Design review of the part built by this model. Coordinates are the model's own, in mm. A direction names the side the tool comes from. Give positions to 0.01 mm unless a question says otherwise; leave off trailing zeros. Write each loop counter-clockwise with the first axis right and the second up, starting at its lowest first coordinate (ties: lowest second). Pieces come first, ordered by that corner, then holes. Notation, with made-up numbers: (-0.75, 41) -> (32.25, 41) arc R22 ccw to (32.25, 67) -> close; hole circle Ø11 at (80.5, 68). An arc over 180 degrees is marked (long way). Write each question's results on one line, items separated by ' | '. Start each with the question number.
(1) Take a section at D-D (x = -28). State the section outline as (y, z) points (3 decimals).
(2) To check wall thickness, follow probe 1 along Z at (x, y) = (-16.5, -0.7); probe 2 along Z at (x, y) = (-2, -0.65); probe 3 along X at (y, z) = (-0.5, -3). State the ranges of each line that lie inside material, in increasing order.
(3) Mouldability with a two-part tool opening along Z and no side actions: class faces 3 (the face through (6, -3.175, -3)), 4 (the face through (-8.774, -1.565, -53.198)), 5 (the face through (-5.525, -1.565, 3.131)) as released by +Z, released by -Z, zero draft, split by the parting line, or undercut.
(4) Clearance check with flat-ended pins moving along their axes: pin 1 (1 mm diameter, centred on x = 24, y = -1.5, fed in from -Z); pin 2 (1 mm diameter, centred on x = -1.5, y = -2, fed in from +Z); pin 3 (6 mm diameter, centred on x = -46, z = 6.5, fed in from +Y). State where each tip first meets the part, or that it passes through.
(5) For faces 1 (the face through (5.474, -1.565, 3.219)), 2 (the face through (6, 0, -3)), list the 3-axis set-ups (+Z, -Z, +X, -X, +Y, -Y) from which the entire face can be reached by the end or side of a thin tool; tool diameter is ignored.
(6) Take a section at B-B (z = -13). State the section outline as (x, y) points (3 decimals), plus the area to 3 significant figures.
(7) Take a section at A-A (y = -2.2). State the section outline as (x, z) points, plus the area to 3 significant figures.
(8) Take a section at C-C (z = 18). State the section outline as (x, y) points (3 decimals), plus the area to 3 significant figures.
from build123d import *

# Parameters (mm, degrees)
F1_DEPTH = 3.175


with BuildPart() as f1:
    # F0 (on Front) → F1 (new body)
    with BuildSketch(Plane.XZ):
        with BuildLine():
            ThreePointArc((32.9955675162, -19.0500006373), (36.8017738864, -9.8610059738), (38.1, 0))
            ThreePointArc((38.1, 0), (26.9407683703, 26.9407683561), (2.01e-08, 38.1))
            ThreePointArc((2.01e-08, 38.1), (-32.9955680289, 19.0499997494), (-32.9955675847, -19.0500005187))
            ThreePointArc((-32.9955675847, -19.0500005187), (-6.85e-08, -38.1), (32.9955675162, -19.0500006373))
        make_face()
        Polygon((3.6661742094, 6.35), (7.3323484187, 0), (3.6661742094, -6.35), (-3.6661742094, -6.35), (-7.3323484187, 0), (-3.6661742094, 6.35), align=None, mode=Mode.SUBTRACT)
        with BuildLine():
            ThreePointArc((2.01e-08, 38.1), (26.9407683703, 26.9407683561), (38.1, 0))
            ThreePointArc((38.1, 0), (36.8017738864, -9.8610059738), (32.9955675162, -19.0500006373))
            ThreePointArc((32.9955675162, -19.0500006373), (40.6079799838, -0.6720115922), (43.2044321158, 19.05))
            ThreePointArc((43.2044321158, 19.05), (43.1497599719, 21.9360086092), (42.9858219927, 24.8178758988))
            ThreePointArc((42.9858219927, 24.8178758988), (22.4955313049, 34.7037847321), (2.01e-08, 38.1))
        make_face()
        with BuildLine():
            ThreePointArc((-32.9955675847, -19.0500005187), (-32.9955680289, 19.0499997494), (2.01e-08, 38.1))
            ThreePointArc((2.01e-08, 38.1), (-22.4955312856, 34.703784738), (-42.9858219927, 24.8178758988))
            ThreePointArc((-42.9858219927, 24.8178758988), (-41.3021247691, 2.1298089138), (-32.9955675847, -19.0500005187))
        make_face()
        with BuildLine():
            ThreePointArc((-42.9858219927, 24.8178758988), (-22.4955312856, 34.703784738), (2.01e-08, 38.1))
            ThreePointArc((2.01e-08, 38.1), (-21.6006695494, 53.4773083041), (-14.1409580475, 78.92142827))
            ThreePointArc((-14.1409580475, 78.92142827), (-34.2450737922, 54.8987950557), (-42.9858219927, 24.8178758988))
        make_face()
        with BuildLine():
            ThreePointArc((0, -49.6357517976), (18.8065932705, -36.833594191), (32.9955675162, -19.0500006373))
            ThreePointArc((32.9955675162, -19.0500006373), (-6.85e-08, -38.1), (-32.9955675847, -19.0500005187))
            ThreePointArc((-32.9955675847, -19.0500005187), (-18.8065933208, -36.8335941444), (0, -49.6357517976))
        make_face()
        with BuildLine():
            ThreePointArc((43.2044321158, 19.05), (40.6079799838, -0.6720115922), (32.9955675162, -19.0500006373))
            ThreePointArc((32.9955675162, -19.0500006373), (57.1130420252, -8.0319255321), (75.4184408331, -27.2142854025))
            ThreePointArc((75.4184408331, -27.2142854025), (64.6662880971, 2.2077062576), (42.9858219927, 24.8178758988))
            ThreePointArc((42.9858219927, 24.8178758988), (43.1497599719, 21.9360086092), (43.2044321158, 19.05))
        make_face()
        with BuildLine():
            ThreePointArc((0, -49.6357517976), (-18.8065933208, -36.8335941444), (-32.9955675847, -19.0500005187))
            ThreePointArc((-32.9955675847, -19.0500005187), (-30.7118441482, -24.5633969182), (-29.9329086147, -30.48))
            ThreePointArc((-29.9329086147, -30.48), (-39.9745190131, -49.4079816151), (-61.2774832447, -51.7071428447))
            ThreePointArc((-61.2774832447, -51.7071428447), (-30.4212145195, -57.1065013952), (0, -49.6357517976))
        make_face()
    extrude(amount=F1_DEPTH)


solid = f1.part
Report:
1) outline: (-3.175, -56.986) -> (0, -56.986) -> (0, 64.723) -> (-3.175, 64.723) -> close
2) probe 1: -55.34 to 45.14, 76.78 to 76.99 | probe 2: -50.56 to -6.35, 6.35 to 38.19 | probe 3: -39.94 to -5.6, 5.6 to 67.63
3) face 3: zero draft | face 4: released by -Z | face 5: undercut
4) pin 1: z = -32.08 | pin 2: z = 38.19 | pin 3: through
5) face 1: +Y, -Y | face 2: +Z, -Z, +X, -X, +Y
6) outline: (-36.136, -3.175) -> (38.061, -3.175) -> (38.061, 0) -> (-36.136, 0) -> close; (67.525, -3.175) -> (71.947, -3.175) -> (71.947, 0) -> (67.525, 0) -> close | area: 250 mm2
7) outline: (-61.28, -51.71) arc R76.2 ccw to (33, -19.05) arc R22.86 cw to (75.42, -27.21) arc R76.2 ccw to (0, 38.1) arc R22.86 cw to (-14.14, 78.92) arc R76.2 ccw to (-33, -19.05) arc R22.86 cw to start; hole (-7.33, 0) -> (-3.67, -6.35) -> (3.67, -6.35) -> (7.33, 0) -> (3.67, 6.35) -> (-3.67, 6.35) -> close | area: 7,340 mm2
8) outline: (-43.197, -3.175) -> (51.568, -3.175) -> (51.568, 0) -> (-43.197, 0) -> close | area: 301 mm2
